The model under review builds one solid part; all positions refer to its coordinate system, in mm. A direction names the side the tool comes from. Coordinates: 2 decimals unless noted, no trailing zeros. Order: outer loops, then holes, each group sorted by start corner. A loop starts at its lowest first (then second) coordinate and runs counter-clockwise, first axis right, second up. Notation, with made-up numbers: (12.5, 18.5) -> (56.5, 18.5) arc R33 cw to (56.5, 47.5) -> close; hole circle Ø11 at (34.5, 13). An arc over 180 degrees is marked (long way). Answer as CSV lines item,"result". Start each with the question number.
Autodesk Inventor part; units mm, degrees
ref_plane "YZ Plane" through (0, 0, 0) normal (1, 0, 0) x (0, 1, 0)
ref_plane "XZ Plane" through (0, 0, 0) normal (0, 1, 0) x (-1, 0, 0)
ref_plane "XY Plane" through (0, 0, 0) normal (0, 0, 1) x (1, 0, 0)
sketch "Boceto1" plane through (0, 0, 0) normal (0, 1, 0) x (-1, 0, 0)
  circle A0 centre (0, 0) radius 27.5
  circle A1 centre (0, 0) radius 25
  circle A2 centre (0, 0) radius 7.5
  arc A3 (1, 1.118) -> (1, -1.118) centre (0, 0) ccw
  line L0 (1, 1.118) -> (1, -1.118)
  dimension "d0" = 55
  dimension "d1" = 50
  dimension "d2" = 15
  dimension "d3" = 3
  dimension "d6" = 1
extrude "Extrusión1" add sketch "Boceto1" along normal mid plane 5
sketch "Boceto2" plane through (0, 0, 0) normal (0, 1, 0) x (-1, 0, 0)
  arc A0 (7.0711, -2.5) -> (7.0711, 2.5) centre (0, 0) ccw
  arc A1 (24.8747, -2.5) -> (24.8747, 2.5) centre (0, 0) ccw
  line L0 (7.0711, 2.5) -> (24.8747, 2.5)
  line L1 (24.8747, -2.5) -> (7.0711, -2.5)
  dimension "d9" = 15
  dimension "d10" = 50
  dimension "d12" = 2.5
extrude "Extrusión2" add sketch "Boceto2" along normal mid plane 3
pattern_circular "Patrón circular1" count 5 over 360 about axis through (0, -10, 0) along (0, 1, 0) of "Extrusión2"
properties part number "Rueda"
1) Tool access review of faces 4 (the face through (13, -1.5, -9)), 5 (the face through (-7.275, -0.021, -14.3)), 6 (the face through (-16, 1.5, 0)), 7 (the face through (1.63, -0.04, 7.32)): name each direction out of +Z, -Z, +X, -X, +Y, -Y from which nothing blocks a thin tool from reaching the whole face with its end or side.
2) Wall thickness on L1, parallel to X at y = -0.35, z = 20; L2, parallel to X at y = -2.3, z = -5; L3, parallel to X at y = 0.5, z = -10.5: over which ranges is each line inside the solid? List them lowest first. Write a range as [from, to].
3) Consider section B-B (x = 23.5). Give the boundary of the cut face in (y, z).
4) Consider section C-C (y = 0.8). Give the boundary of the cut face in (x, z), plus the area to 3 significant figures.
5) Consider section D-D (x = -12). Give the boundary of the cut face in (y, z), plus the area to 3 significant figures.
6) Consider section A-A (z = 0). Give the boundary of the cut face in (x, y), plus the area to 3 significant figures.
7) Mouldability with a two-part tool opening along X and no side actions: class faces 1 (the face through (0, -2.5, -2)), 2 (the face through (5.961, 0.035, -26.846)), 3 (the face through (13, 1.5, 9)) as released by +X, released by -X, zero draft, split by the parting line, or undercut.
8) Insertion check: pin 1 Ø16 at (x, z) = (12.5, -9.5) entering from -Y; pin 2 Ø0.9 at (x, y) = (-16.5, 0.5) entering from -Z; pin 3 Ø11.5 at (x, z) = (-5, 15.5) entering from +Y; pin 4 Ø2 at (x, z) = (9.5, 1) entering from +Y. Each pin has a flat end and moves straight along its axis. Give the tip position at first contact, or say it passes through.
Result:
1,face 4,"-Y"
1,face 5,"+Y, -Y"
1,face 6,"+Y"
1,face 7,"none"
2,L1,"[-18.87, -15], [-9.13, -3.87], [15, 18.87]"
2,L2,"[-27.04, -24.49], [-5.59, 5.59], [24.49, 27.04]"
2,L3,"[-25.42, -22.69], [-6.04, -0.78], [10.2, 18.71], [22.69, 25.42]"
3,outline,"(-2.5, -14.28) -> (2.5, -14.28) -> (2.5, -8.53) -> (-2.5, -8.53) -> close; (-2.5, 8.53) -> (2.5, 8.53) -> (2.5, 14.28) -> (-2.5, 14.28) -> close"
4,outline,"circle Ø55 at (0, 0); hole (-24.87, -2.5) arc R25 ccw to (-10.06, -22.88) -> (-4.56, -5.95) arc R7.5 cw to (-7.07, -2.5) -> close; hole (-24.87, 2.5) -> (-7.07, 2.5) arc R7.5 cw to (-4.56, 5.95) -> (-10.06, 22.88) arc R25 ccw to start; hole (-5.31, -24.43) arc R25 ccw to (18.65, -16.64) -> (4.25, -6.18) arc R7.5 cw to (0.19, -7.5) -> close; hole (-5.31, 24.43) -> (0.19, 7.5) arc R7.5 cw to (4.25, 6.18) -> (18.65, 16.64) arc R25 ccw to start; hole (-1, -1.12) arc R1.5 ccw (long way) to (-1, 1.12) -> close; hole (7.19, -2.13) -> (21.59, -12.6) arc R25 ccw to (21.59, 12.6) -> (7.19, 2.13) arc R7.5 cw to start"
4,area,"1,020 mm2"
5,outline,"(-2.5, -24.74) -> (2.5, -24.74) -> (2.5, -21.93) -> (-2.5, -21.93) -> close; (-2.5, 21.93) -> (2.5, 21.93) -> (2.5, 24.74) -> (-2.5, 24.74) -> close; (-1.5, -2.5) -> (1.5, -2.5) -> (1.5, 2.5) -> (-1.5, 2.5) -> close"
5,area,"43.1 mm2"
6,outline,"(-27.5, -2.5) -> (-25, -2.5) -> (-25, -1.5) -> (-7.5, -1.5) -> (-7.5, -2.5) -> (-1, -2.5) -> (-1, 2.5) -> (-7.5, 2.5) -> (-7.5, 1.5) -> (-25, 1.5) -> (-25, 2.5) -> (-27.5, 2.5) -> close; (1.5, -2.5) -> (7.5, -2.5) -> (7.5, 2.5) -> (1.5, 2.5) -> close; (25, -2.5) -> (27.5, -2.5) -> (27.5, 2.5) -> (25, 2.5) -> close"
6,area,"140 mm2"
7,face 1,"zero draft"
7,face 2,"split by the parting line"
7,face 3,"undercut"
8,pin 1,"y = -1.5"
8,pin 2,"z = -22.33"
8,pin 3,"y = 1.5"
8,pin 4,"through"
